Build history of the part. All positions in model axes, mm. A direction names the side the tool comes from. Give positions to 0.01 mm unless a question says otherwise; leave off trailing zeros. Loops run counter-clockwise (first coordinate to the right, second up) from the corner with the lowest first, then second, coordinate; pieces in that order, holes last. Notation, with made-up numbers: (88, -25.75) - (135, -25.75) arc R13 cw to (135, -11.75) - close; hole circle Ø1 at (23, -25). An arc over 180 degrees is marked (long way). Return JSON: item names as keys, results as strings. Group by question number.
1) Slice it at B-B (x = 0). List the corners of the cut face in (y, z) (3 decimals).
2) Slice it at C-C (z = 1.6). Count the separate pieces of the cut face and the enclosed holes in it, and give its area (3 significant figures).
3) 3-axis set-ups, long thin cutter, end or side, ignore diameter. For faces 1 (the face through (-10, 1, 0)), 2 (the face through (4.762, -25, 2)): which of +Z, -Z, +X, -X, +Y, -Y reach the whole face in a straight line?
4) Mould opens along X. For faces 3 (the face through (0.1, -43.1, 1.6)), 4 (the face through (-28.04, 61.95, 1.61)), 5 (the face through (-10, -62.9, 2)), 6 (the face through (0.1, 7.7, 1.6)) say: released by +X, released by -X, zero draft, split by the parting line, or undercut.
5) Slice it at A-A (y = 53). List the corners of the cut face in (x, z) (3 decimals).
6) Drill centre lines: probe 1 along Y at (x, z) = (0, 0.6); probe 2 along X at (y, z) = (-30.5, 2.2); probe 3 along X at (y, z) = (-53, 2.4). Where is each one in solid material? Low to high. Write a range as from..to.
```python
from build123d import *

# Parameters (mm, degrees)
SKETCH1_W               = 19.800000024
SKETCH1_H               = 125.800000114
SKETCH1_R               = 3.3
SKETCH1_W_2             = 19.05
BOSS_EXTRUDE1_DEPTH     = 3.175
CUT_EXTRUDE1_DEPTH      = 70.315172458
CUT_EXTRUDE1_DEPTH_BACK = 70.315172458
FILLET1_R               = 3.175


with BuildPart() as part:
    # Sketch1 → Boss-Extrude1 (new body)
    # profile 1 of 2: a face of its own
    with BuildSketch(Plane.XY):
        Rectangle(SKETCH1_W, SKETCH1_H)
        with Locations((0, -53.000000045)):
            Circle(SKETCH1_R, mode=Mode.SUBTRACT)
        with Locations((0, 53.000000045)):
            Circle(SKETCH1_R, mode=Mode.SUBTRACT)
    # profile 2 of 2: a face of its own
    with BuildSketch(Plane.XY):
        with Locations((-19.425000012, 0)):
            Rectangle(SKETCH1_W_2, SKETCH1_H)
    extrude(amount=BOSS_EXTRUDE1_DEPTH)

    # Sketch6 → Cut-Extrude1 (cut, two sides: drawn at the far end of the back side and taken through both)
    with BuildSketch(Plane.XY.offset(3.175).offset(-CUT_EXTRUDE1_DEPTH_BACK)):
        with BuildLine():
            Line((4.7625, 38.337500033), (4.7625, 12.462499967))
            ThreePointArc((4.7625, 12.462499967), (0, 7.699999967), (-4.7625, 12.462499967))
            Line((-4.7625, 12.462499967), (-4.7625, 38.337500033))
            ThreePointArc((-4.7625, 38.337500033), (0, 43.100000033), (4.7625, 38.337500033))
        make_face()
        with BuildLine():
            Line((4.7625, -12.462499967), (4.7625, -38.337500033))
            ThreePointArc((4.7625, -38.337500033), (0, -43.100000033), (-4.7625, -38.337500033))
            Line((-4.7625, -38.337500033), (-4.7625, -12.462499967))
            ThreePointArc((-4.7625, -12.462499967), (0, -7.699999967), (4.7625, -12.462499967))
        make_face()
    extrude(amount=CUT_EXTRUDE1_DEPTH + CUT_EXTRUDE1_DEPTH_BACK, mode=Mode.SUBTRACT)

    # Fillet1
    fillet1_edges = [part.edges().sort_by_distance(p)[0] for p in [
        (9.900000012, 62.900000057, 1.5875),
        (9.900000012, -62.900000057, 1.5875),
        (-28.950000012, -62.900000057, 1.5875),
        (-28.950000012, 62.900000057, 1.5875),
    ]]
    fillet(fillet1_edges, radius=FILLET1_R)


solid = part.part
```
Results:
{
 "1": {"outline": "(-62.9, 0) - (-56.3, 0) - (-56.3, 3.175) - (-62.9, 3.175) - close; (-49.7, 0) - (-43.1, 0) - (-43.1, 3.175) - (-49.7, 3.175) - close; (-7.7, 0) - (7.7, 0) - (7.7, 3.175) - (-7.7, 3.175) - close; (43.1, 0) - (49.7, 0) - (49.7, 3.175) - (43.1, 3.175) - close; (56.3, 0) - (62.9, 0) - (62.9, 3.175) - (56.3, 3.175) - close"},
 "2": {"separate pieces": "1", "enclosed holes": "4", "area": "4,170 mm2"},
 "3": {"face 1": "-Z, +X, -X, +Y, -Y", "face 2": "+Z, -Z"},
 "4": {"face 3": "undercut", "face 4": "released by -X", "face 5": "zero draft", "face 6": "undercut"},
 "5": {"outline": "(-28.95, 0) - (-3.3, 0) - (-3.3, 3.175) - (-28.95, 3.175) - close; (3.3, 0) - (9.9, 0) - (9.9, 3.175) - (3.3, 3.175) - close"},
 "6": {"probe 1": "-62.9..-56.3, -49.7..-43.1, -7.7..7.7, 43.1..49.7, 56.3..62.9", "probe 2": "-28.95..-4.76, 4.76..9.9", "probe 3": "-28.95..-3.3, 3.3..9.9"}
}
